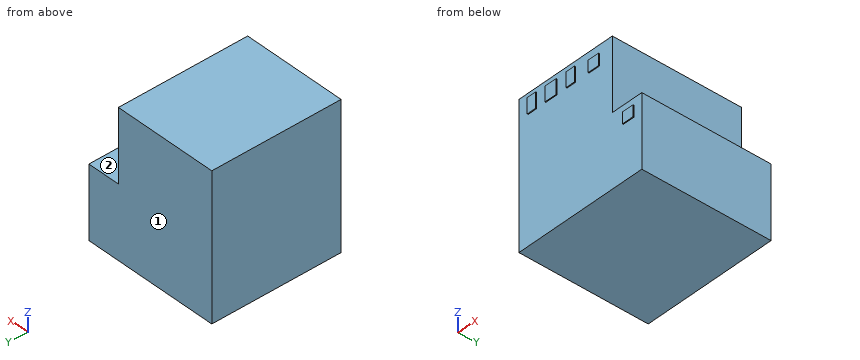
```python
from build123d import *

# Parameters (mm, degrees)
F0_W     = 9.6260905266
F0_H     = 21.1938368157
F1_DEPTH = 12.7
F2_DEPTH = 25.4
F4_W     = 3.3827349544
F4_H     = 3.4457910806
F3_W     = 2.7738437057
F3_H     = 4.3759718537
F3_W_2   = 3.7164986134
F3_H_2   = 4.3712295592
F3_W_3   = 2.7477294207
F3_H_3   = 4.5251846313
F3_W_4   = 3.4826546907
F3_H_4   = 3.3152103424
F5_DEPTH = 0.254


with BuildPart() as f1:
    # F0 (on Front) → F1 (new body)
    with BuildSketch(Plane.XZ):
        Polygon((-85.2284654975, 24.0949820727), (-115.7357469201, 24.0949820727), (-115.7357469201, -18.2926915586), (-85.2284654975, -18.2926915586), (-85.2284654975, 2.9011452571), align=None)
        with Locations((-80.4154202342, -7.6957731508)):
            Rectangle(F0_W, F0_H)
    extrude(amount=F1_DEPTH)

    # F2 (add): a face of the model
    f2_faces = [f1.faces().sort_by_distance(p)[0] for p in [
        (-97.7476505301, -12.7, 1.4571198832),
    ]]
    extrude(f2_faces, amount=F2_DEPTH)

    # F4 (on face) + F3 (on face) → F5 (join)
    with BuildSketch(Plane.XZ.offset(38.1)):
        with Locations((-91.1433510482, 19.9342770502)):
            Rectangle(F4_W, F4_H)
    with BuildSketch(Plane.XZ.offset(38.1)):
        with Locations((-98.6624695361, 20.3993674368)):
            Rectangle(F3_W, F3_H)
        with Locations((-105.1291897893, 20.3969962895)):
            Rectangle(F3_W_2, F3_H_2)
        with Locations((-111.3641187549, 20.4739738256)):
            Rectangle(F3_W_3, F3_H_3)
        with Locations((-79.9321979284, -0.7592802867)):
            Rectangle(F3_W_4, F3_H_4)
    extrude(amount=F5_DEPTH)


solid = f1.part
```
Source: CAD feature listing. Evaluate the final solid. Frame: model axes, mm. Face numbers are marked on the shaded views. A direction names the side the tool comes from. Round coordinates to 2 decimals unless told otherwise and drop trailing zeros. Loops run counter-clockwise (first coordinate to the right, second up) from the corner with the lowest first, then second, coordinate; pieces in that order, holes last. Notation, with made-up numbers: M 57.5,15.25 L 98.5,15.25 A24 cw 98.5,29.25 Z; hole C 48,61 d1. An arc over 180 degrees is marked long. Use a Markdown table: item, result. Add a question column.
1. Ray query, line 1 along Y through (x, z) = (-89, 9.5); line 2 along X through (y, z) = (-14, 12.5); line 3 along Z through (x, y) = (-79, -23). Return the intervals inside material, ascending. Write a range as [from, to].
2. Cut plane C-C, the plane z = 3.5. Output: boundary loops of the cut face in (x, y).
3. Cut plane B-B, the plane x = -81. Output: boundary loops of the cut face in (y, z), and give its area (3 significant figures).
4. Contact query for flat-ended pins moving along their axis: pin 1 (2 mm diameter, centred on x = -80, z = 4.5, fed in from -Y); pin 2 (1 mm diameter, centred on x = -111, z = -12, fed in from -Y); pin 3 (6.5 mm diameter, centred on y = -12, z = 10.5, fed in from +X). Output: stop coordinate, or through.
5. Cut plane A-A, the plane y = -29. Output: boundary loops of the cut face in (x, z), and give its area (3 significant figures).
6. Set-up query: the marked faces 1 and 2. Return all of +Z, -Z, +X, -X, +Y, -Y with unobstructed straight access to the full face (end or side cutting, diameter ignored); none if empty.
Solution:
| question | item | result |
|---|---|---|
| 1 | line 1 | y = [-38.1, 0] |
| 1 | line 2 | x = [-115.74, -85.23] |
| 1 | line 3 | z = [-18.29, 2.9] |
| 2 | outline | M -115.74,-38.1 L -85.23,-38.1 L -85.23,0 L -115.74,0 Z |
| 3 | outline | M -38.35,-2.42 L -38.1,-2.42 L -38.1,-18.29 L 0,-18.29 L 0,2.9 L -38.1,2.9 L -38.1,0.9 L -38.35,0.9 Z |
| 3 | area | 808 mm2 |
| 4 | pin 1 | passes through |
| 4 | pin 2 | stops at y = -38.1 |
| 4 | pin 3 | stops at x = -85.23 |
| 5 | outline | M -115.74,-18.29 L -75.6,-18.29 L -75.6,2.9 L -85.23,2.9 L -85.23,24.09 L -115.74,24.09 Z |
| 5 | area | 1,500 mm2 |
| 6 | face 1 | +Z, -Z, +X, -X, +Y |
| 6 | face 2 | +Z, +X, +Y, -Y |
